Input: part model. Units: mm. Frame: model coordinates. Face numbers are marked on the shaded views. A direction names the side the tool comes from. Round coordinates to 2 decimals unless told otherwise and drop trailing zeros. Write each loop counter-clockwise with the first axis right and the second up, starting at its lowest first coordinate (ties: lowest second). Pieces come first, ordered by that corner, then holes. Notation, with made-up numbers: (52.25, 53.5) -> (88.25, 53.5) arc R27 cw to (88.25, 88.5) -> close; hole circle Ø7 at (52, 19.5). An arc over 180 degrees is marked (long way). Use CSV: the item, a comma, the result in double quotes.
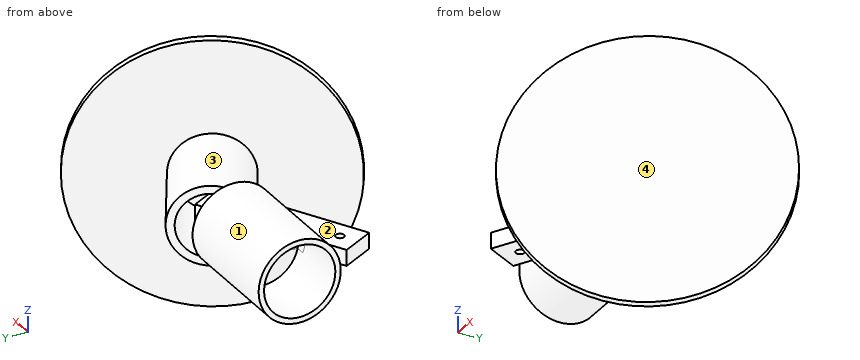
```python
from build123d import *
from build123d.topology import SkipClean

# Parameters (mm, degrees)
TAB_DEPTH               = 3
CABLE_PIN_HOLE_SKETCH_R = 1.6
CABLE_PIN_HOLE_DEPTH    = 6
BORE_CLEAR_SKETCH_W     = 26
BORE_CLEAR_SKETCH_H     = 13.45


with BuildPart() as part:
    # Pad And Pedestal Sketch → Pad And Pedestal (revolve)
    with BuildSketch(Plane.XY):
        Polygon((1481.589408105, -12.415318093), (1506.420044292, 30.983293711), (1503.816127584, 32.473131883), (1486.434682253, 2.094103619), (1455.187681754, 19.972161674), (1453.697843582, 17.368244965), (1482.340927374, 0.980025082), (1476.381574689, -9.435641751), align=None)
    revolve(axis=Axis((1511.968436369, -29.796763424, 0), (-0.8679722360942783, 0.4966127237289622, 0)))

    # Socket Sketch → Socket (revolve)
    with BuildSketch(Plane.XY, mode=Mode.PRIVATE) as socket_sk:
        Polygon((1400, 13.45), (1400, 15.5), (1444.890102203, 15.5), (1444.890102203, 10), (1430, 10), (1430, 0), (1425, 0), (1425, 13.45), align=None)
    revolve(socket_sk.sketch.rotate(Axis((-3000, 0, 0), (1, 0, 0)), 90), axis=Axis((-3000, 0, 0), (1, 0, 0)))

    # Tab Sketch → Tab (add, symmetric)
    with BuildSketch(Plane.XY):
        Polygon((1465.019568481, -5.166098693), (1413.342666954, -33.635342599), (1406.587253146, -21.373026982), (1458.264154673, 7.096216924), align=None)
    extrude(amount=TAB_DEPTH, both=True)

    # Cable Pin Hole Sketch → Cable Pin Hole (cut, symmetric)
    with BuildSketch(Plane.XY):
        with Locations(Location((1416.096117858, -24.126477887, 0), (0, 0, 180))):
            Circle(CABLE_PIN_HOLE_SKETCH_R)
    extrude(amount=CABLE_PIN_HOLE_DEPTH, both=True, mode=Mode.SUBTRACT)

    # Bore Clear Sketch → Bore Clear (revolve, cut)
    with SkipClean():  # the faces are left unmerged after this step: merging them gives an invalid solid
        with BuildSketch(Plane.XY):
            with Locations((1412, 6.725)):
                Rectangle(BORE_CLEAR_SKETCH_W, BORE_CLEAR_SKETCH_H)
        revolve(axis=Axis((-3000, 0, 0), (1, 0, 0)), mode=Mode.SUBTRACT)
    add(part.part.scale(1), mode=Mode.REPLACE)  # the faces are merged on a copy


solid = part.part
```
Item 1: Line query: line 1 (Y direction, x = 1405.75, z = 0); line 2 (Y direction, x = 1407.5, z = 0); line 3 (X direction, y = 14, z = 8). Output: solid intervals per line, ascending.
Worked answers:
line 1,"y = -15.5 to -13.45, 13.45 to 15.5"
line 2,"y = -23.03 to -20.87, -15.5 to -13.45, 13.45 to 15.5"
line 3,"x = 1453.43 to 1460.97, 1493.25 to 1496.7"
Item 2: Set-up query: the marked faces 1 and 2. Return all of +Z, -Z, +X, -X, +Y, -Y with unobstructed straight access to the full face (end or side cutting, diameter ignored); none if empty.
Worked answers:
face 1,"-X"
face 2,"none"
Item 3: Section query A-A on x = 1432. Return the cut outline in (y, z).
Worked answers:
outline,"(-23.36, -3) -> (-15.21, -3) arc R15.5 ccw (long way) to (-15.21, 3) -> (-23.36, 3) -> close; hole (-9.54, -3) arc R10 ccw (long way) to (-9.54, 3) -> (-7.37, 3) -> (-7.37, -3) -> close"
Item 4: Pull-direction query (X, two-part tool) for the marked faces 3 and 4; classes: +X half, -X half, draft (parallel to the pull), parting line (faces both ways), or undercut.
Worked answers:
face 3,"undercut"
face 4,"+X half"
Item 5: Section query C-C on z = -23.5. Return the cut outline in (x, y), plus the area to 3 significant figures.
Worked answers:
outline,"(1457.07, -49.23) -> (1459.67, -50.72) -> (1503.51, 25.89) -> (1500.9, 27.38) -> close"
area,"265 mm²"
Item 6: Section query B-B on z = 32.5. Return the cut outline in (x, y).
Worked answers:
outline,"(1460.12, -43.91) -> (1462.72, -45.4) -> (1500.46, 20.56) -> (1497.86, 22.05) -> close"
Item 7: First-contact query: pin 1 Ø10 at (y, z) = (2, 1) entering from +X; pin 2 Ø3 at (x, z) = (1457, 15) entering from -Y; pin 3 Ø24 at (y, z) = (0, 0) entering from +X; pin 4 Ø4 at (x, y) = (1474, -33) entering from -Z. Flat tips, straight axial feed; report the tip coordinate or a pass-through.
Worked answers:
pin 1,"stops at x = 1492.7"
pin 2,"stops at y = -54.16"
pin 3,"stops at x = 1495.56"
pin 4,"passes through"
